Autodesk Fusion 360 part; units mm, degrees
sketch "Sketch1" plane through (0, 0, 0) normal (0, 0, 1) x (1, 0, 0)
  circle A0 centre (0, 0) radius 17.5
  dimension "d1" = 35
ref_plane "WorkPlane1" through (0, 0, 20) normal (0, 0, 1) x (1, 0, 0)
sketch "Sketch2" plane through (0, 0, 20) normal (0, 0, 1) x (1, 0, 0)
  circle A0 centre (0, 0) radius 16
  dimension "d3" = 32
loft "Loft1" add profiles "Sketch1", "Sketch2" section 1 section 2
ref_plane "WorkPlane2" through (0, 0, 10) normal (0, 0, 1) x (1, 0, 0)
sketch "Sketch3" plane through (0, 0, 10) normal (0, 0, 1) x (1, 0, 0)
  circle A0 centre (0, 0) radius 7.5
  dimension "d5" = 15
sketch "Sketch4" plane through (0, 0, 20) normal (0, 0, 1) x (-1, 0, 0)
  circle A0 centre (0, 0) radius 16
  circle A1 centre (0, 0) radius 9
  dimension "d6" = 18
loft "Loft2" cut profiles "Sketch3", "Sketch4" section 1 section 2 contours A1
fillet "Fillet1" radius 2.3 2 edges at (8.3909, -3.2545, 20) (-14.9172, 5.7858, 20)
sketch "Sketch5" plane through (0, 0, 10) normal (0, 0, 1) x (-1, 0, 0)
  circle A0 centre (0, 0) radius 7.5
  circle A1 centre (0, 0) radius 4.575
  dimension "d9" = 9.15
extrude "Extrude1" cut sketch "Sketch5" against normal blind 10 contours A1
sketch "Sketch6" plane through (0, 0, 10) normal (0, 0, 1) x (-1, 0, 0)
  circle A0 centre (0, 0) radius 4.575
  circle A1 centre (0, 0) radius 7.5
  circle A2 centre (0, 0) radius 7.15
  dimension "d12" = 14.3
extrude "Extrude2" cut sketch "Sketch6" against normal blind 5 contours A2
equation "d4 = -20 mm + 10 mm"
Read the model definition and answer for the solid it produces. Units are mm, in the model's axes. A direction names the side the tool comes from. Coordinates: 2 decimals unless noted, no trailing zeros. Order: outer loops, then holes, each group sorted by start corner. A loop starts at its lowest first (then second) coordinate and runs counter-clockwise, first axis right, second up. Notation, with made-up numbers: (39.25, 75) - (78.25, 75) arc R13 cw to (78.25, 98) - close; hole circle Ø4 at (82, 13). An arc over 180 degrees is marked (long way). Answer as a JSON object with one key per item and string values. Group by question number.
Item 1: A tool of negligible diameter and unlimited length cuts with its end or side. For faces 1 (the face through (-2.459, -3.858, 2.535)), 2 (the face through (0, 5, 5)), from which of +Z, -Z, +X, -X, +Y, -Y can it reach the whole face along a straight path? Write none if from no direction.
Item 2: Section C-C (z = 9) is taken. Give the vertices of the cut face in (x, y) (3 decimals).
Item 3: The mould has two halves that part along Y. Classify faces 3 (the face through (0.93, -7.09, 7.54)), 4 (the face through (-4.17, 10.34, 20)), 5 (the face through (15.92, -5.01, 10.8)): +Y half, -Y half, draft (parallel to the pull), parting line (faces both ways), or undercut.
Item 4: Section A-A (x = 0) is taken. Give the vertices of the cut face in (y, z) (3 decimals).
Item 5: Flat-ended cylindrical pins translate along their axes: P1, Ø1.5, axis at y = -2, z = 14.5, coming from the +X side; P2, Ø16.5, axis at x = 0.5, y = 1.5, coming from the +Z side; P3, Ø1.5, axis at y = 5, z = 14, coming from the +X side. Find the tip coordinate at first contact, or state that the pin passes through.
Item 6: Consider probe 1 along X at (y, z) = (0, 7.2); probe 2 along Y at (x, z) = (0, 8.3); probe 3 along Y at (x, z) = (-1.5, 8.25). Determine where each line is inside the solid, lowest interval first. Write a range as from..to.
Results are:
{
 "1": {"face 1": "+Z, -Z", "face 2": "+Z"},
 "2": {"outline": "circle Ø33.65 at (0, 0); hole circle Ø14.3 at (0, 0)"},
 "3": {"face 3": "undercut", "face 4": "draft", "face 5": "parting line"},
 "4": {"outline": "(-17.5, 0) - (-4.575, 0) - (-4.575, 5) - (-7.15, 5) - (-7.15, 10) - (-7.5, 10) - (-8.706, 18.041) arc R2.3 ccw to (-10.981, 20) - (-13.866, 20) arc R2.3 ccw to (-16.16, 17.872) - close; (4.575, 0) - (17.5, 0) - (16.16, 17.872) arc R2.3 ccw to (13.866, 20) - (10.981, 20) arc R2.3 ccw to (8.706, 18.041) - (7.5, 10) - (7.15, 10) - (7.15, 5) - (4.575, 5) - close"},
 "5": {"P1": "stops at x = 16.39", "P2": "stops at z = 19.69", "P3": "stops at x = 15.9"},
 "6": {"probe 1": "x = -16.96..-7.15, 7.15..16.96", "probe 2": "y = -16.88..-7.15, 7.15..16.88", "probe 3": "y = -16.81..-6.99, 6.99..16.81"}
}
